from build123d import *

# Parameters (mm, degrees)
F0_W     = 50
F0_H     = 150
F0_R     = 5.5
F1_DEPTH = 2.5


with BuildPart() as f1:
    # F0 (on Front) → F1 (new body, symmetric)
    with BuildSketch(Plane.XZ):
        Rectangle(F0_W, F0_H)
        with Locations((0, -50)):
            Circle(F0_R, mode=Mode.SUBTRACT)
        with Locations((0, 50)):
            Circle(F0_R, mode=Mode.SUBTRACT)
    extrude(amount=F1_DEPTH, both=True)


solid = f1.part
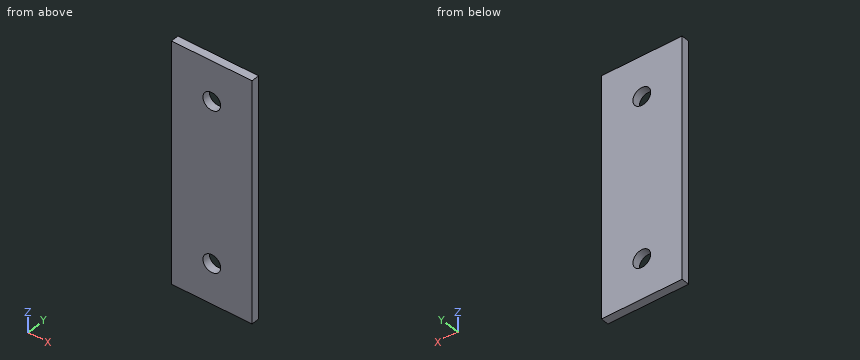
Verification items for the finished model (mm, model axes). Round coordinates to 2 decimals unless told otherwise and drop trailing zeros. Loops run counter-clockwise (first coordinate to the right, second up) from the corner with the lowest first, then second, coordinate; pieces in that order, holes last. Notation, with made-up numbers: M -17.5,-35 L 41.5,-35 A18 cw 41.5,-6 Z; hole C 82,-2 d10. An arc over 180 degrees is marked long. Write each question's results on one line, items separated by ' | '.
1) Section check A-A on z = 50. Record the boundary of the cut face in (x, y).
Checks:
outline: M -25,-2.5 L -5.5,-2.5 L -5.5,2.5 L -25,2.5 Z; M 5.5,-2.5 L 25,-2.5 L 25,2.5 L 5.5,2.5 Z
2) Scan line: L1, parallel to Z at x = 0, y = -1.45. Record every from-to range of solid material in increasing order. Write a range as from..to.
Checks:
L1: z = -75..-55.5, -44.5..44.5, 55.5..75
3) Section check B-B on x = 0. Record the boundary of the cut face in (y, z).
Checks:
outline: M -2.5,-75 L 2.5,-75 L 2.5,-55.5 L -2.5,-55.5 Z; M -2.5,-44.5 L 2.5,-44.5 L 2.5,44.5 L -2.5,44.5 Z; M -2.5,55.5 L 2.5,55.5 L 2.5,75 L -2.5,75 Z
4) Section check C-C on y = 1.15. Record the boundary of the cut face in (x, z), then the cut area to 3 significant figures.
Checks:
outline: M -25,-75 L 25,-75 L 25,75 L -25,75 Z; hole C 0,-50 d11; hole C 0,50 d11 | area: 7,310 mm2
